Read the model definition and answer for the solid it produces. Units are mm, in the model's axes. Face numbers are marked on the shaded views. A direction names the side the tool comes from. Coordinates: 2 decimals unless noted, no trailing zeros. Order: outer loops, then holes, each group sorted by start corner. A loop starts at its lowest first (then second) coordinate and runs counter-clockwise, first axis right, second up. Notation, with made-up numbers: (68, 15.25) - (106, 15.25) arc R15 ccw to (106, 29.25) - close; hole circle Ø10 at (60.25, -25). An arc over 180 degrees is marked (long way). Use one line per item in the form item = value. Start each with the question number.
from build123d import *

# Parameters (mm, degrees)
F1_DEPTH = 18.5
F2_R     = 7.25
F3_DEPTH = 18.501


with BuildPart() as f1:
    # F0 (on Front) → F1 (new body)
    with BuildSketch(Plane.XZ):
        Polygon((7.794229, 13.5), (-7.794229, 13.5), (-15.588457, 0), (-7.794229, -13.5), (7.794229, -13.5), (15.588457, 0), align=None)
    extrude(amount=F1_DEPTH)

    # F2 (on face) → F3 (cut, through all)
    with BuildSketch(Plane.XZ.offset(18.5)):
        Circle(F2_R)
    extrude(amount=-F3_DEPTH, mode=Mode.SUBTRACT)

    # F4 (on Right) → F5 (revolve, cut)
    with BuildSketch(Plane.YZ):
        Polygon((-16.25, 0), (0, 0), (0, 11.577), (-7.5, 11.577), (-7.5, 12), (-16.25, 12), align=None)
    revolve(axis=Axis((0, -8.125, 0), (0, 1, 0)), mode=Mode.SUBTRACT)


solid = f1.part
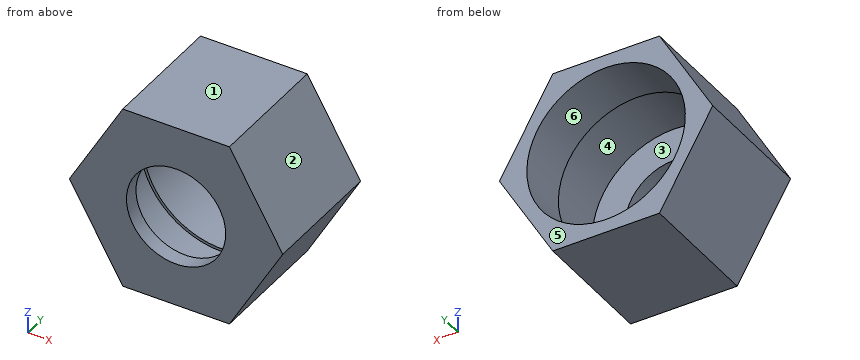
Q1. A cutting plane is placed at C-C (z = -1.5). Give the vertices of the cut face in (x, y).
Q2. For a pull along X with two mould halves and no side action, classify the marked faces 1, 2, 3 and 4 as +X half, -X half, draft (parallel to the pull), parting line (faces both ways), or undercut.
Q3. Which of the six approach directions +Z, -Z, +X, -X, +Y, -Y give full straight-line access (tool end or side, diameter ignored) to the marked faces 5 and 6?
Q4. A cutting plane is placed at B-B (y = -10.75). Give the vertices of the cut face in (x, z), then the cut area to 3 significant figures.
Q5. A cutting plane is placed at A-A (x = 0). Give the vertices of the cut face in (y, z), then the cut area to 3 significant figures.
Q6. Given P1, Ø6, axis at y = -16, z = -1, coming from the -X side; P2, Ø1, axis at y = -9.5, z = -2, coming from the -X side; P3, Ø11.5, axis at x = 0, z = 0, coming from the -Y side; P4, Ø6, axis at y = -9, z = 10.5, coming from the +X side, each flat-ended and moving along its own axis, determine where each tip first touches the part or whether it passes through.
Q7. A cutting plane is placed at D-D (x = 10). Give the vertices of the cut face in (y, z).
Q8. Consider probe 1 along X at (y, z) = (-11, 0); probe 2 along Z at (x, y) = (0, -17.8); probe 3 along X at (y, z) = (-1.75, 0). Determine where each line is inside the solid, lowest interval first.
Result sheet:
q1.outline = (-14.72, -18.5) - (-7.09, -18.5) - (-7.09, -16.25) - (-11.91, -16.25) - (-11.91, -7.5) - (-11.48, -7.5) - (-11.48, 0) - (-14.72, 0) - close; (7.09, -18.5) - (14.72, -18.5) - (14.72, 0) - (11.48, 0) - (11.48, -7.5) - (11.91, -7.5) - (11.91, -16.25) - (7.09, -16.25) - close
q2.face_1 = draft
q2.face_2 = +X half
q2.face_3 = undercut
q2.face_4 = undercut
q3.face_5 = +Z, -Z, +X, -X, +Y
q3.face_6 = +Y
q4.outline = (-15.59, 0) - (-7.79, -13.5) - (7.79, -13.5) - (15.59, 0) - (7.79, 13.5) - (-7.79, 13.5) - close; hole circle Ø24 at (0, 0)
q4.area = 179 mm^2
q5.outline = (-18.5, -13.5) - (0, -13.5) - (0, -11.58) - (-7.5, -11.58) - (-7.5, -12) - (-16.25, -12) - (-16.25, -7.25) - (-18.5, -7.25) - close; (-18.5, 7.25) - (-16.25, 7.25) - (-16.25, 12) - (-7.5, 12) - (-7.5, 11.58) - (0, 11.58) - (0, 13.5) - (-18.5, 13.5) - close
q5.area = 83.2 mm^2
q6.P1 = -15.59
q6.P2 = -14.72
q6.P3 = through
q6.P4 = 11.26
q7.outline = (-18.5, -9.68) - (0, -9.68) - (0, -5.83) - (-7.5, -5.83) - (-7.5, -6.63) - (-16.25, -6.63) - (-16.25, 6.63) - (-7.5, 6.63) - (-7.5, 5.83) - (0, 5.83) - (0, 9.68) - (-18.5, 9.68) - close
q8.probe_1 = -15.59 to -12, 12 to 15.59
q8.probe_2 = -13.5 to -7.25, 7.25 to 13.5
q8.probe_3 = -15.59 to -11.58, 11.58 to 15.59
